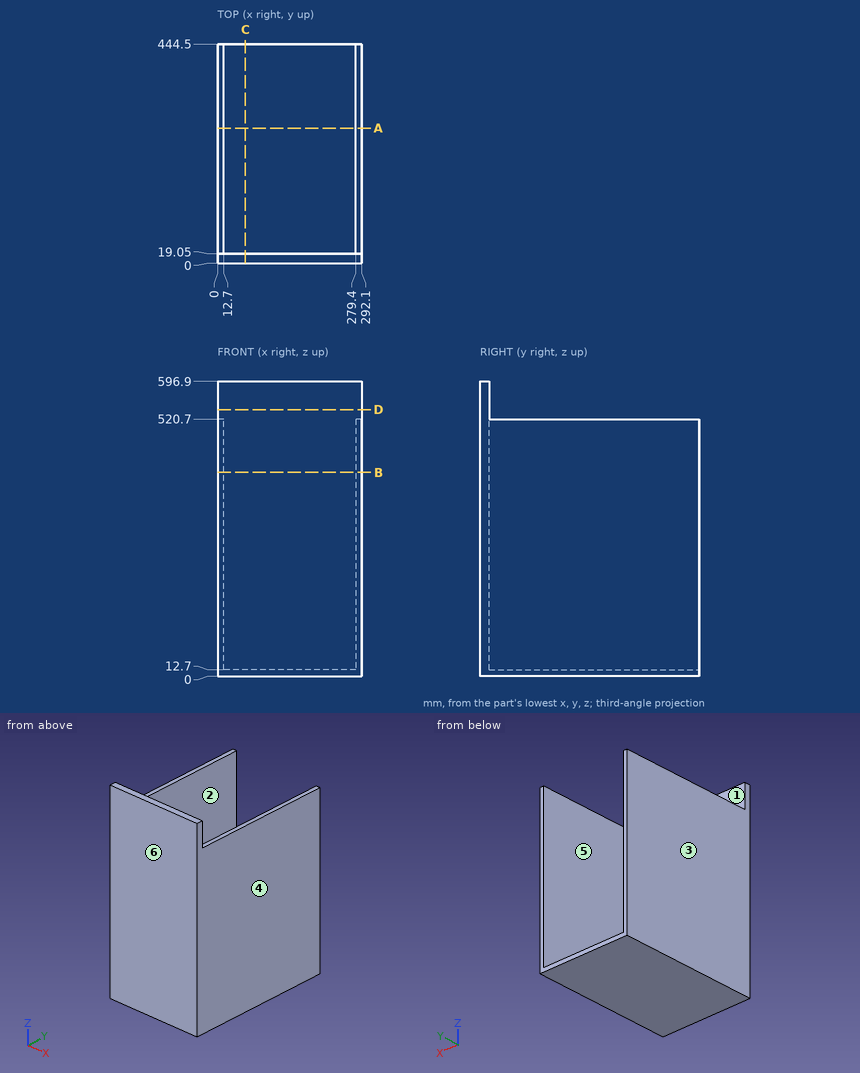
Geometry: see drawing. Coordinates: mm, zero at the bounding-box minimum. A direction names the side the tool comes from. Coordinates: 2 decimals unless noted, no trailing zeros. Order: outer loops, then holes, each group sorted by start corner. A loop starts at its lowest first (then second) coordinate and runs counter-clockwise, first axis right, second up. Notation, with made-up numbers: (19.25, 84.5) - (39.25, 84.5) arc R7 cw to (39.25, 90.5) - close; hole circle Ø1 at (79, -14). An arc over 180 degrees is marked (long way). Write each question's results on one line, items separated by ' | '.
(1) Line query: line 1 (X direction, y = 74, z = 75); line 2 (Y direction, x = 57, z = 396); line 3 (Z direction, x = 207.5, y = 417.5). Output: solid intervals per line, ascending. Write a range as [from, to].
Values found:
line 1: x = [0, 12.7], [279.4, 292.1] | line 2: y = [0, 19.05] | line 3: z = [0, 12.7]
(2) Section query C-C, the plane x = 56. Return the cut outline in (y, z).
Values found:
outline: (0, 0) - (444.5, 0) - (444.5, 12.7) - (19.05, 12.7) - (19.05, 596.9) - (0, 596.9) - close
(3) Section query D-D, the plane z = 539.5. Return the cut outline in (x, y), plus the area to 3 significant figures.
Values found:
outline: (0, 0) - (292.1, 0) - (292.1, 19.05) - (0, 19.05) - close | area: 5,560 mm²
(4) First-contact query: pin 1 Ø1 at (x, z) = (105, 213) entering from -Y; pin 2 Ø5 at (x, y) = (54.5, 300) entering from +Z; pin 3 Ø2 at (x, z) = (82.5, 448.5) entering from +Y; pin 4 Ø6.5 at (x, y) = (282.5, 274.5) entering from +Z. Flat tips, straight axial feed; report the tip coordinate or a pass-through.
Values found:
pin 1: stops at y = 0 | pin 2: stops at z = 12.7 | pin 3: stops at y = 19.05 | pin 4: stops at z = 520.7
(5) Section query B-B, the plane z = 412.5. Return the cut outline in (x, y).
Values found:
outline: (0, 0) - (292.1, 0) - (292.1, 444.5) - (279.4, 444.5) - (279.4, 19.05) - (12.7, 19.05) - (12.7, 444.5) - (0, 444.5) - close
(6) Mould query, pull axis X, two halves, no side actions, for the marked faces 1, 2, 3 and 4. Classes: +X half, -X half, draft (parallel to the pull), parting line (faces both ways), or undercut.
Values found:
face 1: undercut | face 2: undercut | face 3: -X half | face 4: +X half
(7) Section query A-A, the plane y = 274. Return the cut outline in (x, z), plus the area to 3 significant figures.
Values found:
outline: (0, 0) - (292.1, 0) - (292.1, 520.7) - (279.4, 520.7) - (279.4, 12.7) - (12.7, 12.7) - (12.7, 520.7) - (0, 520.7) - close | area: 16,600 mm²
(8) Set-up query: the marked faces 5 and 6. Return all of +Z, -Z, +X, -X, +Y, -Y with unobstructed straight access to the full face (end or side cutting, diameter ignored); none if empty.
Values found:
face 5: +Z, +Y | face 6: +Z, -Z, +X, -X, -Y
